Geometry: final body of the model. Coordinates: model frame, mm. Coordinates: 2 decimals unless noted, no trailing zeros. Write each loop counter-clockwise with the first axis right and the second up, starting at its lowest first coordinate (ties: lowest second). Pieces come first, ordered by that corner, then holes. Notation, with made-up numbers: (77.25, -37.5) -> (95.25, -37.5) arc R18 ccw to (95.25, -28.5) -> close; hole circle Ø6 at (49, 13). An arc over 180 degrees is marked (long way). One line per item, written item: value.
```python
from build123d import *

# Parameters (mm, degrees)
SKETCH1_R                   = 70
SKETCH1_R_2                 = 30
SKETCH1_R_3                 = 3
SKETCH1_W                   = 2
SKETCH1_H                   = 5
SKETCH1_W_2                 = 22.5
SKETCH1_H_2                 = 12
SKETCH1_W_3                 = 5
SKETCH1_H_3                 = 2
Y_KSEKLIK_EKSTR_ZYON1_DEPTH = 2


with BuildPart() as part:
    # Sketch1 → Yükseklik-Ekstrüzyon1 (new body)
    with BuildSketch(Plane(origin=(0, 0, 0), x_dir=(1, 0, 0), z_dir=(0, 1, 0))):
        with Locations(Location((0, 0, 0), (0, 0, 270))):
            Circle(SKETCH1_R)
        with Locations(Location((0, 0, 0), (0, 0, 270))):
            Circle(SKETCH1_R_2, mode=Mode.SUBTRACT)
        with Locations(Location((39.748737342, 0, 0), (0, 0, 270))):
            Circle(SKETCH1_R_3, mode=Mode.SUBTRACT)
        with Locations(Location((-39.748737342, 0, 0), (0, 0, 270))):
            Circle(SKETCH1_R_3, mode=Mode.SUBTRACT)
        with Locations(Location((0, 39.748737342, 0), (0, 0, 270))):
            Circle(SKETCH1_R_3, mode=Mode.SUBTRACT)
        with Locations((-29, 27.5)):
            Rectangle(SKETCH1_W, SKETCH1_H, mode=Mode.SUBTRACT)
        with Locations((29, 27.5)):
            Rectangle(SKETCH1_W, SKETCH1_H, mode=Mode.SUBTRACT)
        with Locations((-29, -27.5)):
            Rectangle(SKETCH1_W, SKETCH1_H, mode=Mode.SUBTRACT)
        with Locations((29, -27.5)):
            Rectangle(SKETCH1_W, SKETCH1_H, mode=Mode.SUBTRACT)
        with Locations((-39.748737342, 39.748737342)):
            Rectangle(SKETCH1_W, SKETCH1_H, mode=Mode.SUBTRACT)
        with Locations((39.748737342, 39.748737342)):
            Rectangle(SKETCH1_W, SKETCH1_H, mode=Mode.SUBTRACT)
        with Locations((39.748737342, -39.748737342)):
            Rectangle(SKETCH1_W, SKETCH1_H, mode=Mode.SUBTRACT)
        with Locations((-39.748737342, -39.748737342)):
            Rectangle(SKETCH1_W, SKETCH1_H, mode=Mode.SUBTRACT)
        with Locations((0, -39.748737342)):
            Rectangle(SKETCH1_W_2, SKETCH1_H_2, mode=Mode.SUBTRACT)
        with Locations((-64.748737342, 4)):
            Rectangle(SKETCH1_W_3, SKETCH1_H_3, mode=Mode.SUBTRACT)
        with Locations((-64.748737342, -4)):
            Rectangle(SKETCH1_W_3, SKETCH1_H_3, mode=Mode.SUBTRACT)
        with Locations((-54.748737342, -4)):
            Rectangle(SKETCH1_W_3, SKETCH1_H_3, mode=Mode.SUBTRACT)
        with Locations((-54.748737342, 4)):
            Rectangle(SKETCH1_W_3, SKETCH1_H_3, mode=Mode.SUBTRACT)
        with Locations((-4, 64.748737342)):
            Rectangle(SKETCH1_W, SKETCH1_H, mode=Mode.SUBTRACT)
        with Locations((-4, 54.748737342)):
            Rectangle(SKETCH1_W, SKETCH1_H, mode=Mode.SUBTRACT)
        with Locations((4, 54.748737342)):
            Rectangle(SKETCH1_W, SKETCH1_H, mode=Mode.SUBTRACT)
        with Locations((4, 64.748737342)):
            Rectangle(SKETCH1_W, SKETCH1_H, mode=Mode.SUBTRACT)
        with Locations((54.748737342, 4)):
            Rectangle(SKETCH1_W_3, SKETCH1_H_3, mode=Mode.SUBTRACT)
        with Locations((54.748737342, -4)):
            Rectangle(SKETCH1_W_3, SKETCH1_H_3, mode=Mode.SUBTRACT)
        with Locations((64.748737342, 4)):
            Rectangle(SKETCH1_W_3, SKETCH1_H_3, mode=Mode.SUBTRACT)
        with Locations((64.748737342, -4)):
            Rectangle(SKETCH1_W_3, SKETCH1_H_3, mode=Mode.SUBTRACT)
        with Locations((-4, -54.748737342)):
            Rectangle(SKETCH1_W, SKETCH1_H, mode=Mode.SUBTRACT)
        with Locations((4, -54.748737342)):
            Rectangle(SKETCH1_W, SKETCH1_H, mode=Mode.SUBTRACT)
        with Locations((4, -64.748737342)):
            Rectangle(SKETCH1_W, SKETCH1_H, mode=Mode.SUBTRACT)
        with Locations((-4, -64.748737342)):
            Rectangle(SKETCH1_W, SKETCH1_H, mode=Mode.SUBTRACT)
    extrude(amount=Y_KSEKLIK_EKSTR_ZYON1_DEPTH)


solid = part.part
```
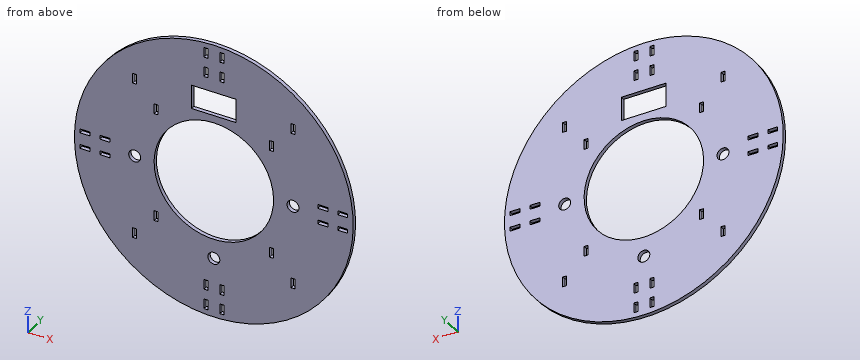
(1) Line query: line 1 (X direction, y = 1.45, z = 0); line 2 (X direction, y = 0.7, z = -4.5); line 3 (Z direction, x = -64, y = 0.5). Output: solid intervals per line, ascending. Write a range as [from, to].
Responses:
line 1: x = [-70, -42.75], [-36.75, -30], [30, 36.75], [42.75, 70]
line 2: x = [-69.86, -67.25], [-62.25, -57.25], [-52.25, -29.66], [29.66, 52.25], [57.25, 62.25], [67.25, 69.86]
line 3: z = [-28.35, -5], [-3, 3], [5, 28.35]
(2) Section A-A (z = 0). Return the cut outline in (x, y).
Responses:
outline: (-70, 0) -> (-42.75, 0) -> (-42.75, 2) -> (-70, 2) -> close; (-36.75, 0) -> (-30, 0) -> (-30, 2) -> (-36.75, 2) -> close; (30, 0) -> (36.75, 0) -> (36.75, 2) -> (30, 2) -> close; (42.75, 0) -> (70, 0) -> (70, 2) -> (42.75, 2) -> close
(3) Section B-B (x = 0). Return the cut outline in (y, z).
Responses:
outline: (0, -70) -> (2, -70) -> (2, -42.75) -> (0, -42.75) -> close; (0, -36.75) -> (2, -36.75) -> (2, -30) -> (0, -30) -> close; (0, 30) -> (2, 30) -> (2, 33.75) -> (0, 33.75) -> close; (0, 45.75) -> (2, 45.75) -> (2, 70) -> (0, 70) -> close
(4) Section C-C (x = -17.5). Return the cut outline in (y, z), then the cut area to 3 significant figures.
Responses:
outline: (0, -67.78) -> (2, -67.78) -> (2, -24.37) -> (0, -24.37) -> close; (0, 24.37) -> (2, 24.37) -> (2, 67.78) -> (0, 67.78) -> close
area: 174 mm2
(5) First-contact query: pin 1 (1 mm diameter, centred on y = 1, z = 3.5, fed in from +X); pin 2 (0.6 mm diameter, centred on x = 29, y = 1, fed in from +Z); pin 3 (1 mm diameter, centred on x = 14.5, y = 1.5, fed in from +Z). Flat tips, straight axial feed; report the tip coordinate or a pass-through.
Responses:
pin 1: stops at x = 69.94
pin 2: stops at z = 63.85
pin 3: stops at z = 68.59
(6) Section D-D (z = -16.5). Return the cut outline in (x, y).
Responses:
outline: (-68.03, 0) -> (-25.05, 0) -> (-25.05, 2) -> (-68.03, 2) -> close; (25.05, 0) -> (68.03, 0) -> (68.03, 2) -> (25.05, 2) -> close
